The listing builds one solid part. Answer for the finished solid, in the listing's coordinates (mm). A direction names the side the tool comes from. Coordinates: 2 decimals unless noted, no trailing zeros. Order: outer loops, then holes, each group sorted by start corner. A loop starts at its lowest first (then second) coordinate and runs counter-clockwise, first axis right, second up. Notation, with made-up numbers: (35, -25.75) -> (70, -25.75) arc R22 ccw to (70, 2.25) -> close; hole circle Ø9 at (5.5, 68). An arc over 180 degrees is marked (long way). Return JSON: item names as keys, results as strings.
```python
from build123d import *

# Parameters (mm, degrees)
F0_R     = 5.5
F1_DEPTH = 3
F2_R     = 4
F3_DEPTH = 30
F4_W     = 0.9
F4_H     = 0.5
F6_SIZE  = 0.5


with BuildPart() as f1:
    # F0 (on Right) → F1 (new body)
    with BuildSketch(Plane.YZ):
        Circle(F0_R)
    extrude(amount=-F1_DEPTH)

    # F2 (on face) → F3 (join)
    with BuildSketch(Plane(origin=(-3, 0, 0), x_dir=(0, -1, 0), z_dir=(-1, 0, 0))):
        Circle(F2_R)
    extrude(amount=F3_DEPTH)

    # F4 (on Front) → F5 (revolve, cut)
    with BuildSketch(Plane.XZ):
        with Locations((-13.45, 3.75)):
            Rectangle(F4_W, F4_H)
    revolve(axis=Axis((-16.22575, 0, 0), (1, 0, 0)), mode=Mode.SUBTRACT)

    # F6
    f6_edges = [f1.edges().sort_by_distance(p)[0] for p in [
        (-33, 4, 0),
    ]]
    chamfer(f6_edges, length=F6_SIZE)


solid = f1.part
```
Item 1: Which of the six approach directions +Z, -Z, +X, -X, +Y, -Y give full straight-line access (tool end or side, diameter ignored) to faces 1 (the flat face through (-3, -4, -2)), 2 (the flat face through (0, 0, 0)), 3 (the cylindrical face through (-13.444, 1.341, 3.233))?
Answer list:
{"face 1": "-X", "face 2": "+Z, -Z, +X, +Y, -Y", "face 3": "none"}
Item 2: Flat-ended cylindrical pins translate along their axes: pin 1 (2 mm diameter, centred on x = -22.5, z = -2.5, fed in from +Y); pin 2 (6.5 mm diameter, centred on y = -1.5, z = -1.5, fed in from +X); pin 3 (5 mm diameter, centred on x = -23, z = 3.5, fed in from -Y); pin 4 (4 mm diameter, centred on x = -23, y = 1.5, fed in from +Z). Find the tip coordinate at first contact, or state that the pin passes through.
Answer list:
{"pin 1": "y = 3.71", "pin 2": "x = 0", "pin 3": "y = -3.87", "pin 4": "z = 4"}
Item 3: The part is cut by section D-D on y = -4.5. Determine the outline of the cut face in (x, z).
Answer list:
{"outline": "(-3, -3.16) -> (0, -3.16) -> (0, 3.16) -> (-3, 3.16) -> close"}
Item 4: The part is cut by section A-A on y = 0. Determine the outline of the cut face in (x, z).
Answer list:
{"outline": "(-33, -3.5) -> (-32.5, -4) -> (-13.9, -4) -> (-13.9, -3.5) -> (-13, -3.5) -> (-13, -4) -> (-3, -4) -> (-3, -5.5) -> (0, -5.5) -> (0, 5.5) -> (-3, 5.5) -> (-3, 4) -> (-13, 4) -> (-13, 3.5) -> (-13.9, 3.5) -> (-13.9, 4) -> (-32.5, 4) -> (-33, 3.5) -> close"}
Item 5: The part is cut by section C-C on x = -25.5. Determine the outline of the cut face in (y, z), plus the area to 3 significant figures.
Answer list:
{"outline": "circle Ø8 at (0, 0)", "area": "50.3 mm2"}
Item 6: Find the intervals of material crossed by probe 1 along X at (y, z) = (-5, 0.75); probe 2 along X at (y, z) = (-3.75, 0); probe 3 along Z at (x, y) = (-1.5, -1), in increasing order.
Answer list:
{"probe 1": "-3 to 0", "probe 2": "-32.75 to -13.9, -13 to 0", "probe 3": "-5.41 to 5.41"}
